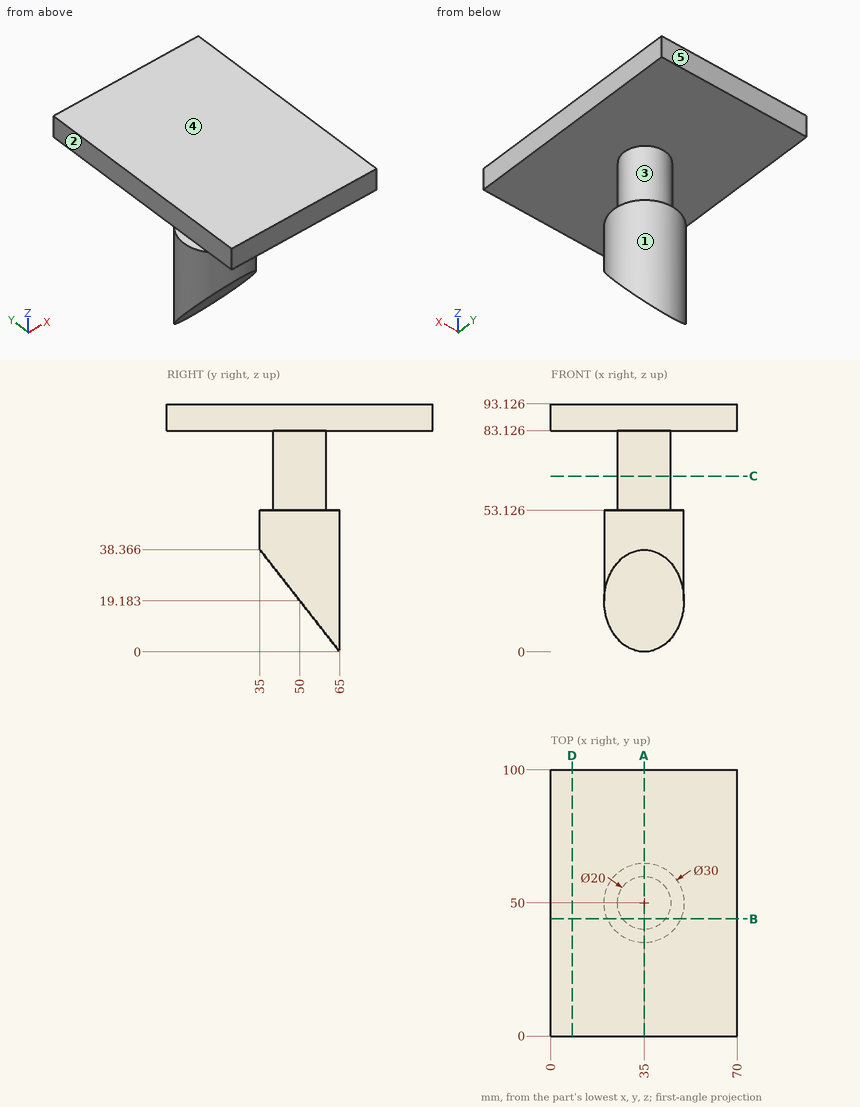
Check sheet for the drawn part. Datum: minimum x, y, z corner. Units: mm. A direction names the side the tool comes from. Give positions to 0.01 mm unless a question says otherwise; leave off trailing zeros. Order: outer loops, then holes, each group sorted by start corner. A loop starts at its lowest first (then second) coordinate and runs counter-clockwise, first axis right, second up. Notation, with made-up numbers: (41.5, 32) -> (86.5, 32) arc R15 cw to (86.5, 36) -> close; hole circle Ø3 at (-11.75, 34.5). An arc over 180 degrees is marked (long way). One line per item, written item: value.
(1) Sectioned sample at B-B on y = 44. Record the cut outline in (x, z) (1 decimal).
Final values:
outline: (0, 83.1) -> (27, 83.1) -> (27, 53.1) -> (21.3, 53.1) -> (21.3, 26.9) -> (48.7, 26.9) -> (48.7, 53.1) -> (43, 53.1) -> (43, 83.1) -> (70, 83.1) -> (70, 93.1) -> (0, 93.1) -> close
(2) Scan lines: line 1 along Z through (x, y) = (29, 7.5) (1 decimal); line 2 along X through (y, z) = (50.5, 51); line 3 along Y through (x, z) = (34.5, 57.5). Record each from-to range of solid material in increasing order. Write a range as [from, to].
Final values:
line 1: [83.1, 93.1]
line 2: [20.01, 49.99]
line 3: [40.01, 59.99]
(3) Tool access check on the marked faces 1 and 2. Record the directions out of +Z, -Z, +X, -X, +Y, -Y that give a thin tool (end or side, any length) a straight path to the whole face; none if there is none.
Final values:
face 1: -Z
face 2: +Z, -Z, -X, +Y, -Y
(4) Draft check along Z on the marked faces 3, 4 and 5. Enter one of: pulls with the +Z half, pulls with the -Z half, needs draft (parallel to the pull), parting line crosses it, or undercut.
Final values:
face 3: undercut
face 4: pulls with the +Z half
face 5: needs draft
(5) Sectioned sample at D-D on x = 8. Record the cut outline in (y, z) (1 decimal), then the cut area to 3 significant figures.
Final values:
outline: (0, 83.1) -> (100, 83.1) -> (100, 93.1) -> (0, 93.1) -> close
area: 1,000 mm^2
(6) Sectioned sample at A-A on x = 35. Record the cut outline in (y, z) (1 decimal), then the cut area to 3 significant figures.
Final values:
outline: (0, 83.1) -> (40, 83.1) -> (40, 53.1) -> (35, 53.1) -> (35, 38.4) -> (65, 0) -> (65, 53.1) -> (60, 53.1) -> (60, 83.1) -> (100, 83.1) -> (100, 93.1) -> (0, 93.1) -> close
area: 2,620 mm^2
(7) Sectioned sample at C-C on z = 66. Record the cut outline in (x, y), then the cut area to 3 significant figures.
Final values:
outline: circle Ø20 at (35, 50)
area: 314 mm^2
(8) Gauge pin test, flat ends, axial feed: pin 1 (5 mm diameter, centred on x = 31, y = 63, fed in from -Z) (1 decimal); pin 2 (1.5 mm diameter, centred on x = 21.5, z = 22.5, fed in from +Y); pin 3 (12 mm diameter, centred on y = 21, z = 72, fed in from +X); pin 4 (5 mm diameter, centred on x = 57, y = 77, fed in from -Z). Record the tip position at first contact, or that the pin passes through.
Final values:
pin 1: z = 0.2
pin 2: y = 57.9
pin 3: through
pin 4: z = 83.13
